Here's how the part is built. I have some questions about the finished solid (model axes, mm). A direction names the side the tool comes from. Give positions to 0.01 mm unless a question says otherwise; leave off trailing zeros. Write each loop counter-clockwise with the first axis right and the second up, starting at its lowest first coordinate (ties: lowest second). Pieces come first, ordered by that corner, then holes. Notation, with made-up numbers: (85, 19.5) -> (127, 19.5) arc R24 ccw to (127, 37.5) -> close; hole circle Ø3 at (-18, 31). An arc over 180 degrees is marked (long way). Put each result on its own line as item: value. Start each with the question number.
from build123d import *

# Parameters (mm, degrees)
SKETCH1_W            = 76.2
SKETCH1_H            = 38.1
SKETCH1_R            = 3.3274
BOSS_EXTRUDE1_DEPTH  = 7.62
SKETCH2_R            = 3.175
BOSS_EXTRUDE2_DEPTH  = 7.62
FILLET1_R            = 7.62
SKETCH3_R            = 6.35
CUT_EXTRUDE1_DEPTH   = 3.81
FILLET1_OF_MIRROR2_R = 7.62


with BuildPart() as part:
    # Sketch1 → Boss-Extrude1 (new body)
    with BuildSketch(Plane(origin=(0, 0, 0), x_dir=(1, 0, 0), z_dir=(0, 1, 0))):
        with Locations((38.1, 19.05)):
            Rectangle(SKETCH1_W, SKETCH1_H)
        with Locations(Location((19.05, 19.05, 0), (0, 0, 90))):
            Circle(SKETCH1_R, mode=Mode.SUBTRACT)
        with Locations(Location((57.15, 19.05, 0), (0, 0, 90))):
            Circle(SKETCH1_R, mode=Mode.SUBTRACT)
    extrude(amount=BOSS_EXTRUDE1_DEPTH)

    # Sketch2 → Boss-Extrude2 (add)
    with BuildSketch(Plane.XY):
        with BuildLine():
            Line((19.05, 7.62), (19.05, 59.69))
            ThreePointArc((19.05, 59.69), (38.1, 78.74), (57.15, 59.69))
            Line((57.15, 59.69), (57.15, 7.62))
            Line((57.15, 7.62), (19.05, 7.62))
        make_face()
        with Locations((38.1, 59.69)):
            Circle(SKETCH2_R, mode=Mode.SUBTRACT)
    boss_extrude2 = extrude(amount=-BOSS_EXTRUDE2_DEPTH)

    # Fillet1
    fillet1_edges = [part.edges().sort_by_distance(p)[0] for p in [
        (38.1, 7.62, -7.62),
        (57.15, 7.62, -3.81),
        (19.05, 7.62, -3.81),
    ]]
    fillet(fillet1_edges, radius=FILLET1_R)

    # Sketch3 → Cut-Extrude1 (cut)
    with BuildSketch(Plane(origin=(0, 0, -7.62), x_dir=(-1, 0, 0), z_dir=(0, 0, -1))):
        with Locations((-38.1, 59.69)):
            Circle(SKETCH3_R)
    cut_extrude1 = extrude(amount=-CUT_EXTRUDE1_DEPTH, mode=Mode.SUBTRACT)

    # Mirror2: Boss-Extrude2, Cut-Extrude1 across plane
    add(boss_extrude2.mirror(Plane.XY.offset(-19.05)))
    add(cut_extrude1.mirror(Plane.XY.offset(-19.05)), mode=Mode.SUBTRACT)

    # Fillet1 of Mirror2
    fillet1_of_mirror2_edges = [part.edges().sort_by_distance(p)[0] for p in [
        (38.1, 7.62, -30.48),
        (57.15, 7.62, -34.29),
        (19.05, 7.62, -34.29),
    ]]
    fillet(fillet1_of_mirror2_edges, radius=FILLET1_OF_MIRROR2_R)


solid = part.part
1) I'm going to push flat-ended pins straight in: pin 1 Ø4 at (y, z) = (39.5, -5.5) entering from -X; pin 2 Ø4 at (y, z) = (20, -8.5) entering from +X; pin 3 Ø5 at (y, z) = (15.5, -9.5) entering from -X. Where does each tip first touch, or does it pass through?
2) I want a section at C-C, the plane z = -5. Write out the boundary of the cut face in (x, y), and give its area (3 significant figures).
3) I want a section at B-B, the plane y = 34. Write out the boundary of the cut face in (x, z).
4) I want a section at D-D, the plane x = 48.5. Write out the boundary of the cut face in (y, z), and give its area (3 significant figures).
5) I want a section at A-A, the plane z = -19.05. Write out the boundary of the cut face in (x, y).
6) Thinking about a two-plate mould opening in Y: for faces 4 (the flat face through (38, 7.62, -21)), 5 (the flat face through (38, 0, -19)), 6 (the flat face through (38, 30, 0)), 7 (the flat face through (37, 63, -3.81)), which applies, released by +Y, released by -Y, zero draft, split by the parting line, or undercut?
7) I need wall thicknesses on probe 1 along X at (y, z) = (4, -19); probe 2 along Z at (x, y) = (40.5, 35); probe 3 along Z at (x, y) = (57.15, 2). Which ranges of each line are inside material? Lowest first, please.
8) Which directions (+Z, -Z, +X, -X, +Y, -Y) give clear straight access to the entire face, cutting with the end or side of a thin tool? Please do faces 1 (the flat face through (57.15, 38, -34)), 2 (the flat face through (37, 63, -34.29)), 3 (the flat face through (19.05, 37, -34)).
Established:
1. pin 1: stops at x = 19.05
1. pin 2: stops at x = 57.15
1. pin 3: stops at x = 18.89
2. outline: (0, 0) -> (76.2, 0) -> (76.2, 7.62) -> (64.77, 7.62) arc R7.62 cw to (57.15, 15.24) -> (57.15, 59.69) arc R19.05 ccw to (19.05, 59.69) -> (19.05, 15.24) arc R7.62 cw to (11.43, 7.62) -> (0, 7.62) -> close; hole circle Ø12.7 at (38.1, 59.69)
2. area: 3,030 mm2
3. outline: (19.05, -38.1) -> (57.15, -38.1) -> (57.15, -30.48) -> (19.05, -30.48) -> close; (19.05, -7.62) -> (57.15, -7.62) -> (57.15, 0) -> (19.05, 0) -> close
4. outline: (0, -38.1) -> (75.65, -38.1) -> (75.65, -30.48) -> (15.24, -30.48) arc R7.62 cw to (7.62, -22.86) -> (7.62, -15.24) arc R7.62 cw to (15.24, -7.62) -> (75.65, -7.62) -> (75.65, 0) -> (0, 0) -> close
4. area: 1,350 mm2
5. outline: (0, 0) -> (15.72, 0) -> (15.72, 7.62) -> (0, 7.62) -> close; (22.38, 0) -> (53.82, 0) -> (53.82, 7.62) -> (22.38, 7.62) -> close; (60.48, 0) -> (76.2, 0) -> (76.2, 7.62) -> (60.48, 7.62) -> close
6. face 4: released by +Y
6. face 5: released by -Y
6. face 6: zero draft
6. face 7: undercut
7. probe 1: x = 0 to 15.72, 22.38 to 53.82, 60.48 to 76.2
7. probe 2: z = -38.1 to -30.48, -7.62 to 0
7. probe 3: z = -38.1 to -22.38, -15.72 to 0
8. face 1: +Z, -Z, +X, +Y
8. face 2: none
8. face 3: +Z, -Z, -X, +Y
